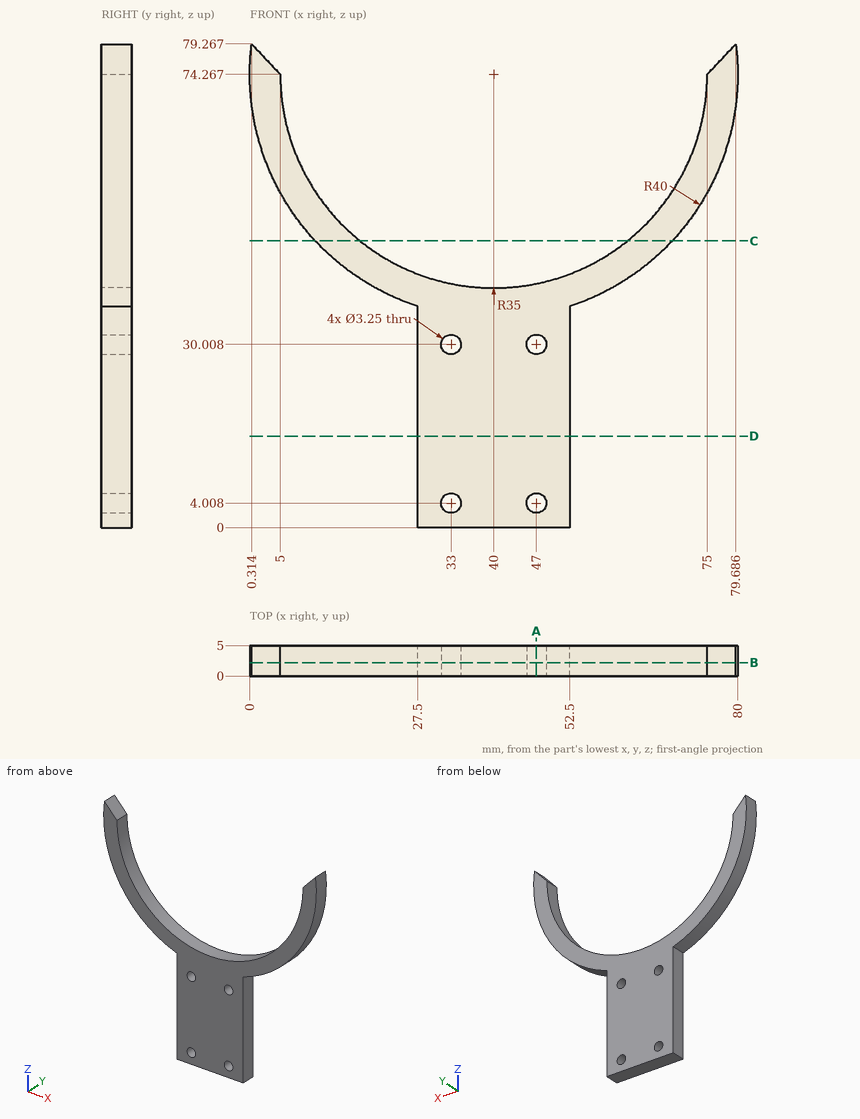
Answer from the drawing. Dimensions are ordinates in mm from the lowest x, y and z of the part. Round coordinates to 2 decimals unless told otherwise and drop trailing zeros. Write each loop counter-clockwise with the first axis right and the second up, starting at its lowest first coordinate (ties: lowest second). Pieces come first, ordered by that corner, then holes. Notation, with made-up numbers: (76.5, 87) -> (104.5, 87) arc R11 ccw to (104.5, 107) -> close; hole circle Ø11 at (76, -35). An arc over 180 degrees is marked (long way). Answer in a Markdown table with one row per item. Add a question column.
1) Find section A-A, the plane x = 47. Determine the outline of the cut face in (y, z).
2) Given P1, Ø2.5, axis at x = 33, z = 30.01, coming from the -Y side; P2, Ø2.5, axis at y = 1.5, z = 25.5, coming from the +X side; P3, Ø2.5, axis at y = 3, z = 16, coming from the -X side, each flat-ended and moving along its own axis, determine where each tip first touches the part or whether it passes through.
3) Find section D-D, the plane z = 15. Determine the outline of the cut face in (x, y).
4) Find section B-B, the plane y = 2.2. State how many separate pieces and enclosed holes the cut face has, and give its area (3 significant figures).
5) Consider line 1 (X direction, y = 0.4, z = 4) (1 decimal); line 2 (Z direction, x = 47.5, y = 3.95); line 3 (X direction, y = 0.75, z = 25.5). Determine where each line is inside the solid, lowest interval first.
6) Find section C-C, the plane z = 47. Determine the outline of the cut face in (x, y).
Findings below:
| question | item | result |
|---|---|---|
| 1 | outline | (0, 0) -> (5, 0) -> (5, 2.38) -> (0, 2.38) -> close; (0, 5.63) -> (5, 5.63) -> (5, 28.38) -> (0, 28.38) -> close; (0, 31.63) -> (5, 31.63) -> (5, 39.97) -> (0, 39.97) -> close |
| 2 | P1 | through |
| 2 | P2 | x = 52.5 |
| 2 | P3 | x = 27.5 |
| 3 | outline | (27.5, 0) -> (52.5, 0) -> (52.5, 5) -> (27.5, 5) -> close |
| 4 | separate pieces | 1 |
| 4 | enclosed holes | 4 |
| 4 | area | 1,450 mm² |
| 5 | line 1 | 27.5 to 31.4, 34.6 to 45.4, 48.6 to 52.5 |
| 5 | line 2 | 0 to 2.46, 5.55 to 28.46, 31.55 to 40.08 |
| 5 | line 3 | 27.5 to 52.5 |
| 6 | outline | (10.73, 0) -> (18.06, 0) -> (18.06, 5) -> (10.73, 5) -> close; (61.94, 0) -> (69.27, 0) -> (69.27, 5) -> (61.94, 5) -> close |
